Could you check a few things on this model? Use its own coordinates, in mm. A direction names the side the tool comes from. Coordinates: 2 decimals unless noted, no trailing zeros. Order: outer loops, then holes, each group sorted by start corner. A loop starts at its lowest first (then second) coordinate and runs counter-clockwise, first axis right, second up.
```python
from build123d import *

# Parameters (mm, degrees)
F1_DEPTH = 36
F2_R     = 1.5
F3_DEPTH = 1.6
F4_W     = 3
F4_H     = 17
F5_DEPTH = 3
F6_W     = 1.9588658989
F6_H     = 17
F7_DEPTH = 4
F7_TAPER = 6.2


with BuildPart() as f1:
    # F0 (on Top) → F1 (new body)
    with BuildSketch(Plane.XY):
        with BuildLine():
            Line((0, 16.1580357461), (0, 0))
            Line((0, 0), (5.4, 0))
            Line((5.4, 0), (5.4, 2.4))
            Line((5.4, 2.4), (2.4, 2.4))
            Line((2.4, 2.4), (2.4, 15.3896428953))
            Line((2.4, 15.3896428953), (17.7915743891, 4.6123464831))
            Line((17.7915743891, 4.6123464831), (42.5417641781, 39.9592806968))
            Line((42.5417641781, 39.9592806968), (43.8924032568, 39.9592806968))
            Line((43.8924032568, 39.9592806968), (43.8924032568, 2.4))
            Line((43.8924032568, 2.4), (40.8924032568, 2.4))
            Line((40.8924032568, 2.4), (40.8924032568, 0))
            Line((40.8924032568, 0), (46.2924032568, 0))
            Line((46.2924032568, 0), (46.2924032568, 40.3592806968))
            ThreePointArc((46.2924032568, 40.3592806968), (45.7066168192, 41.7734942591), (44.2924032568, 42.3592806968))
            Line((44.2924032568, 42.3592806968), (42.3335373579, 42.3592806968))
            ThreePointArc((42.3335373579, 42.3592806968), (41.4100401314, 42.1333023631), (40.6952332693, 41.5064335695))
            Line((40.6952332693, 41.5064335695), (17.2021929301, 7.9548948366))
            Line((17.2021929301, 7.9548948366), (3.1471528727, 17.7963398346))
            ThreePointArc((3.1471528727, 17.7963398346), (1.0765027735, 17.9320574124), (0, 16.1580357461))
        make_face()
    extrude(amount=F1_DEPTH)

    # F2 (on face) → F3 (join)
    with BuildSketch(Plane.XZ):
        with BuildLine():
            Line((-7.7767788619, 0), (0, 0))
            Line((0, 0), (0, 36))
            Line((0, 36), (-10.7767788619, 36))
            Line((-10.7767788619, 36), (-10.7767788619, 29.6889703104))
            ThreePointArc((-10.7767788619, 29.6889703104), (-8.1641973062, 24.1021049808), (-7.2681161721, 18))
            ThreePointArc((-7.2681161721, 18), (-8.1641973062, 11.8978950192), (-10.7767788619, 6.3110296896))
            Line((-10.7767788619, 6.3110296896), (-10.7767788619, 3))
            Line((-10.7767788619, 3), (-10.7767788619, 0))
            Line((-10.7767788619, 0), (-7.7767788619, 0))
        make_face()
        with Locations((-7.7767788619, 3)):
            Circle(F2_R, mode=Mode.SUBTRACT)
        with Locations((-7.7767788619, 33)):
            Circle(F2_R, mode=Mode.SUBTRACT)
        Polygon((42.1804301441, 36), (42.1804301441, 0), (46.2169349194, 0), (55.2232211381, 0), (55.2232211381, 36), align=None)
        with Locations((52.2232211381, 3)):
            Circle(F2_R, mode=Mode.SUBTRACT)
        with Locations((52.2232211381, 33)):
            Circle(F2_R, mode=Mode.SUBTRACT)
    extrude(amount=-F3_DEPTH)

    # F4 (on face) → F5 (cut)
    with BuildSketch(Plane(origin=(0, 0, 0), x_dir=(0, -1, 0), z_dir=(-1, 0, 0))):
        with Locations((-11.6580357461, 11.5)):
            Rectangle(F4_W, F4_H)
    extrude(amount=-F5_DEPTH, mode=Mode.SUBTRACT)

    # F6 (on face) → F7 (cut)
    with BuildSketch(Plane(origin=(0, 42.3592806968, 0), x_dir=(-1, 0, 0), z_dir=(0, 1, 0))):
        with Locations((-43.3129703074, 11.5)):
            Rectangle(F6_W, F6_H)
    extrude(amount=-F7_DEPTH, taper=F7_TAPER, mode=Mode.SUBTRACT)


solid = f1.part
```
Item 1: Which directions (+Z, -Z, +X, -X, +Y, -Y) give clear straight access to the entire face, cutting with the end or side of a thin tool? Please do faces 1 (the face through (51, 1.6, 18)), 2 (the face through (5.4, 1, 18)), 3 (the face through (1, 12, 3)).
Item 2: Suppose I cut it at B-B (y = 37.5). List the corners of the cut face in (x, z) for me.
Item 3: Thinking about a two-plate mould opening in X: for faces 4 (the face through (43, 42.359, 28)), 5 (the face through (45.72, 41.76, 17.75)), 6 (the face through (10, 13, 18)), which applies, +X half, -X half, draft (parallel to the pull), parting line (faces both ways), or undercut?
Item 4: Suppose I cut it at D-D (x = -5). List the corners of the cut face in (y, z) for me.
Item 5: I need wall thicknesses on line 1 (X direction, y = 12.5, z = 11.5); line 2 (X direction, y = 13, z = 28.5); line 3 (X direction, y = 11.5, z = 8). Which ranges of each line are inside material? Lowest first, please.
Item 6: Suppose I cut it at C-C (y = 9). List the corners of the cut face in (x, z) for me, and give its area (3 significant figures).
Item 7: For pin 1 Ø0.7 at (y, z) = (1, 23.5) entering from -X; pin 2 Ø1.8 at (x, z) = (-7.78, 3) entering from +Y; pin 3 Ø10.5 at (y, z) = (7.5, 25.5) entering from +X; pin 4 Ø3.5 at (x, z) = (4, 19) entering from +Y, each with a flat end and sliding along its axis, tell me the tip position at first contact or that it passes through.
Item 8: Suppose I cut it at A-A (z = 33). Count the separate pieces of the cut face and the enclosed holes in it, and give its area (3 significant figures).
Geometry results:
1. face 1: +Z, -Z, +X, +Y
1. face 2: +Z, -Z, -Y
1. face 3: -X
2. outline: (37.89, 0) - (40.82, 0) - (40.82, 36) - (37.89, 36) - close; (43.89, 0) - (46.29, 0) - (46.29, 36) - (43.89, 36) - close
3. face 4: draft
3. face 5: +X half
3. face 6: undercut
4. outline: (0, 0) - (1.6, 0) - (1.6, 36) - (0, 36) - close
5. line 1: x = 6.53 to 10.71, 20.38 to 23.31, 43.89 to 46.29
5. line 2: x = 0 to 2.4, 5.81 to 10, 20.73 to 23.66, 43.89 to 46.29
5. line 3: x = 7.95 to 12.14, 19.68 to 22.61, 43.89 to 46.29
6. outline: (0, 0) - (2.4, 0) - (2.4, 36) - (0, 36) - close; (11.53, 0) - (15.71, 0) - (15.71, 36) - (11.53, 36) - close; (17.93, 0) - (20.86, 0) - (20.86, 36) - (17.93, 36) - close; (43.89, 0) - (46.29, 0) - (46.29, 36) - (43.89, 36) - close
6. area: 429 mm2
7. pin 1: stops at x = -8.09
7. pin 2: passes through
7. pin 3: stops at x = 46.29
7. pin 4: stops at y = 18.14
8. separate pieces: 3
8. enclosed holes: 0
8. area: 331 mm2
